Source: CAD feature listing. Evaluate the final solid. Frame: model axes, mm. A direction names the side the tool comes from. Round coordinates to 2 decimals unless told otherwise and drop trailing zeros. Loops run counter-clockwise (first coordinate to the right, second up) from the corner with the lowest first, then second, coordinate; pieces in that order, holes last. Notation, with made-up numbers: M -27,-24 L 9,-24 A11 ccw 9,-19 Z; hole C 38,-40 d3. An arc over 180 degrees is marked long. One line per item, written item: value.
from build123d import *

# Parameters (mm, degrees)
SKETCH_1_R               = 19
EXTRUDE_5_DEPTH          = 45
EXTRUDE_7_DEPTH          = 8
EXTRUDE_8_DEPTH          = 6
CUT_EXTRUDE_2_DEPTH      = 70.304018822
RIB_2_REACH              = 77.904
SKETCH_7_WALL_W          = 186.009693892
SKETCH_7_WALL_H          = 8
SKETCH_9_R               = 12
CUT_EXTRUDE_3_DEPTH      = 76.903604817
CUT_EXTRUDE_5_DEPTH      = 76.903604758
CUT_EXTRUDE_5_DEPTH_BACK = 76.903604758
SKETCH_10_W              = 8
SKETCH_10_H              = 19


with BuildPart() as part:
    # 草图1 → 凸台-拉伸5 (new body)
    with BuildSketch(Plane(origin=(0, 0, 0), x_dir=(1, 0, 0), z_dir=(0, 1, 0))):
        with Locations(Location((0, 0, 0), (0, 0, 90))):
            Circle(SKETCH_1_R)
    extrude(amount=EXTRUDE_5_DEPTH)

    # 草图2 → 凸台-拉伸7 (add)
    with BuildSketch(Plane(origin=(0, 0, 0), x_dir=(1, 0, 0), z_dir=(0, 1, 0))):
        with BuildLine():
            Line((-40, 19), (0, 19))
            Line((0, 19), (0, -19))
            Line((0, -19), (-40, -19))
            ThreePointArc((-40, -19), (-59, 0), (-40, 19))
        make_face()
    extrude(amount=EXTRUDE_7_DEPTH)

    # 草图4 → 凸台-拉伸8 (add)
    with BuildSketch(Plane(origin=(0, 8, 0), x_dir=(1, 0, 0), z_dir=(0, 1, 0))):
        with BuildLine():
            Line((-10, 11), (-55.491933385, 11))
            add(Edge.make_bspline(
                [(-55.491933385, 11), (-60.019399323, 4.706159899), (-60.317992404, -4.540611583), (-55.491933385, -11)],
                knots=[0, 0, 0, 0, 1, 1, 1, 1], degree=3))
            Line((-55.491933385, -11), (-10, -11))
            Line((-10, -11), (-10, 11))
        make_face()
    extrude(amount=EXTRUDE_8_DEPTH)

    # 草图5 → 切除-拉伸2 (cut, through all)
    with BuildSketch(Plane(origin=(0, 14, 0), x_dir=(1, 0, 0), z_dir=(0, 1, 0))):
        with BuildLine():
            Line((-49, 6), (-58.020969044, 6))
            Line((-58.020969044, 6), (-65.909101598, 0.806430717))
            Line((-65.909101598, 0.806430717), (-58.020969044, -6))
            Line((-58.020969044, -6), (-49, -6))
            ThreePointArc((-49, -6), (-43, 0), (-49, 6))
        make_face()
    extrude(amount=-CUT_EXTRUDE_2_DEPTH, mode=Mode.SUBTRACT)

    # 草图7 wall → 筋2 (add, up to next)
    with BuildSketch(Plane(origin=(-28.5, 27, 0), x_dir=(-0.590016589342, -0.807391122258, 0), z_dir=(0.807391122258, -0.590016589342, 0)), mode=Mode.PRIVATE) as rib_2_sk1:
        Rectangle(SKETCH_7_WALL_W, SKETCH_7_WALL_H)
    rib_2_tool1 = extrude(rib_2_sk1.sketch, amount=RIB_2_REACH, mode=Mode.PRIVATE) - part.part
    add(rib_2_tool1.solids().sort_by_distance((-28.5, 27, 0))[0])

    # 草图9 → 切除-拉伸3 (cut, through all)
    with BuildSketch(Plane(origin=(0, 45, 0), x_dir=(1, 0, 0), z_dir=(0, 1, 0))):
        with Locations(Location((0, 0, 0), (0, 0, 270))):
            Circle(SKETCH_9_R)
    extrude(amount=-CUT_EXTRUDE_3_DEPTH, mode=Mode.SUBTRACT)

    # 草图10 → 切除-拉伸5 (cut, two sides: drawn at the far end of the back side and taken through both)
    with BuildSketch(Plane.XY.offset(-CUT_EXTRUDE_5_DEPTH_BACK)):
        with Locations((0, 40.5)):
            Rectangle(SKETCH_10_W, SKETCH_10_H)
    extrude(amount=CUT_EXTRUDE_5_DEPTH + CUT_EXTRUDE_5_DEPTH_BACK, mode=Mode.SUBTRACT)


solid = part.part
1. Pull-direction query (Z, two-part tool) for faces 4 (the face through (-53, 7, -6)), 5 (the face through (0, 31, -15)), 6 (the face through (-27, 22, 4)); classes: released by +Z, released by -Z, zero draft, split by the parting line, or undercut.
Report:
face 4: undercut
face 5: zero draft
face 6: released by +Z
2. Section query C-C (y = 36). Return the cut outline in (x, z), and give its area (3 significant figures).
Report:
outline: M -21.92,-4 L -18.57,-4 A19 ccw -4,-18.57 L -4,-11.31 A12 cw -4,11.31 L -4,18.57 A19 ccw -18.57,4 L -21.92,4 Z; M 4,-18.57 A19 ccw 4,18.57 L 4,11.31 A12 cw 4,-11.31 Z
area: 593 mm2
3. Ray query, line 1 (X direction, y = 10, z = 0); line 2 (Y direction, x = -15.5, z = 11.5); line 3 (Y direction, x = -27, z = 5). Return the intervals inside material, ascending. Write a range as [from, to].
Report:
line 1: x = [-43, -12], [12, 19]
line 2: y = [0, 8]
line 3: y = [0, 14]
4. Section query B-B (x = -8.5). Return the cut outline in (y, z), and give its area (3 significant figures).
Report:
outline: M 0,-19 L 8,-19 L 8,-16.99 L 45,-16.99 L 45,-8.47 L 0,-8.47 Z; M 0,8.47 L 45,8.47 L 45,16.99 L 8,16.99 L 8,19 L 0,19 Z
area: 799 mm2
5. Section query D-D (y = 24). Return the cut outline in (x, z), and give its area (3 significant figures).
Report:
outline: M -30.69,-4 L -18.57,-4 A19 ccw long -18.57,4 L -30.69,4 Z; hole C 0,0 d24
area: 776 mm2
6. Reachability of faces 1 (the face through (-4, 38, -15)), 2 (the face through (-37, 14, -5)), 3 (the face through (16.856, 22.185, -8.767)) from +Z, -Z, +X, -X, +Y, -Y: full face, straight path, thin tool, end or side. Return the list, or none.
Report:
face 1: +Z, -Z, +Y
face 2: -X, +Y
face 3: +Y
7. Section query A-A (z = 0). Return the cut outline in (x, y), and give its area (3 significant figures).
Report:
outline: M -43,0 L -12,0 L -12,45 L -19,45 L -19,40 L -38,14 L -43,14 Z; M 12,0 L 19,0 L 19,45 L 12,45 Z
area: 1,210 mm2
8. Pin query (flat end, axial travel): pin 1 (4 mm diameter, centred on y = 12.5, z = 11.5, fed in from +X); pin 2 (10 mm diameter, centred on x = -54.5, y = 8.5, fed in from +Z); pin 3 (0.8 mm diameter, centred on x = -56.5, z = 9, fed in from -Y); pin 4 (21.5 mm diameter, centred on x = -30, y = 27.5, fed in from -Z). Return the tip coordinate at first contact, or that it passes through.
Report:
pin 1: stops at x = 16.45
pin 2: stops at z = 16.44
pin 3: stops at y = 0
pin 4: stops at z = -4
